Part model, mm, in its own coordinate system. Face numbers are marked on the shaded views. A direction names the side the tool comes from. Round coordinates to 2 decimals unless told otherwise and drop trailing zeros. Loops run counter-clockwise (first coordinate to the right, second up) from the corner with the lowest first, then second, coordinate; pieces in that order, holes last. Notation, with made-up numbers: M -33,43.25 L 2,43.25 A21 cw 2,54.25 Z; hole C 81,89.5 d8. An arc over 180 degrees is marked long. Answer as CSV lines item,"result". Start each with the question number.
Item 1: Band-saw the part on C-C (z = 3.75). Give the cut face in (x, y), and give its area (3 significant figures).
Item 2: Drop a flat-ended pin along its axis: pin 1 Ø1.5 at (x, z) = (0.5, 1.5) entering from +Y. Give the stop position or say it passes through.
Item 3: Mould opens along Z. For the marked faces 3, 4 and 5 say: pulls with the +Z half, pulls with the -Z half, needs draft (parallel to the pull), parting line crosses it, or undercut.
Item 4: Band-saw the part on A-A (y = 17.25). Give the cut face in (x, z).
Item 5: Band-saw the part on B-B (x = 9). Give the cut face in (y, z).
Item 6: Which spindle directions (+Z, -Z, +X, -X, +Y, -Y) get a long thin tool onto all of the face, cutting with end or side? Do the marked faces 1 and 2. Say none if no direction does.
Item 7: Wall check: line 1 (Z direction, x = 8.75, y = 3.75); line 2 (X direction, y = 23.75, z = 2.5); line 3 (Y direction, x = 12.5, z = 2.25). Give the ranges that are in metal, low to high.
Autodesk Inventor part; units mm, degrees
ref_plane "YZ Plane" through (0, 0, 0) normal (1, 0, 0) x (0, 1, 0)
ref_plane "XZ Plane" through (0, 0, 0) normal (0, 1, 0) x (-1, 0, 0)
ref_plane "XY Plane" through (0, 0, 0) normal (0, 0, 1) x (1, 0, 0)
sketch "Skizze1" plane through (0, 0, 0) normal (0, 1, 0) x (-1, 0, 0)
  line L0 (15, 7.5) -> (-15, 7.5)
  line L1 (-15, 7.5) -> (-15, -7.5)
  line L2 (-15, -7.5) -> (15, -7.5)
  line L3 (15, -7.5) -> (15, 7.5)
  point P0 (0, 0)
  dimension "d0" = 15
  dimension "d1" = 30
  dimension "d2" = 15
  dimension "d3" = 7.5
extrude "Extrusion1" add sketch "Skizze1" along normal blind 30
shell "Wandung1" thickness 2 removed faces 1 at (5, 30, 2.5)
properties part number "Servo Hatlerung"
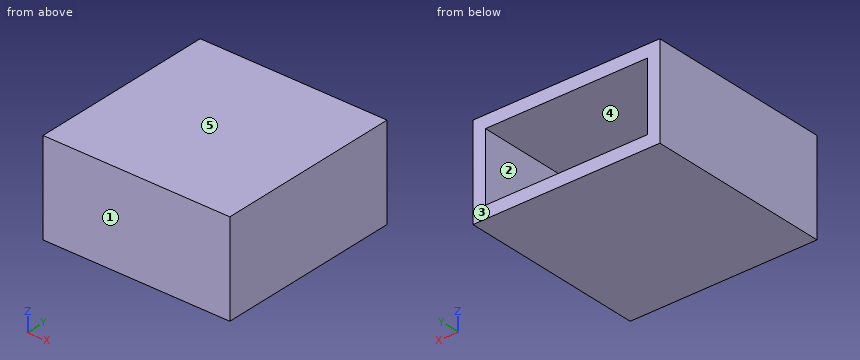
Answer block:
1,outline,"M -15,0 L 15,0 L 15,30 L 13,30 L 13,2 L -13,2 L -13,30 L -15,30 Z"
1,area,"172 mm^2"
2,pin 1,"stops at y = 2"
3,face 3,"needs draft"
3,face 4,"undercut"
3,face 5,"pulls with the +Z half"
4,outline,"M -15,-7.5 L 15,-7.5 L 15,7.5 L -15,7.5 Z; hole M -13,-5.5 L 13,-5.5 L 13,5.5 L -13,5.5 Z"
5,outline,"M 0,-7.5 L 30,-7.5 L 30,-5.5 L 2,-5.5 L 2,5.5 L 30,5.5 L 30,7.5 L 0,7.5 Z"
6,face 1,"+Z, -Z, +X, -X, -Y"
6,face 2,"+Y"
7,line 1,"z = -7.5 to -5.5, 5.5 to 7.5"
7,line 2,"x = -15 to -13, 13 to 15"
7,line 3,"y = 0 to 2"
